Check sheet for the modelled part. Datum: model origin and axes. Units: mm. A direction names the side the tool comes from. Give positions to 0.01 mm unless a question says otherwise; leave off trailing zeros. Loops run counter-clockwise (first coordinate to the right, second up) from the corner with the lowest first, then second, coordinate; pieces in that order, holes last. Notation, with made-up numbers: M 80.5,7 L 119.5,7 A7 ccw 119.5,13 Z; hole C -15.5,76.25 d4. An arc over 180 degrees is marked long. Write each question's results on one line, items separated by ' | '. Start each with the question number.
1. Draft check along Y on faces 4 (the flat face through (59, 0, -65)), 5 (the cylindrical face through (149.01, 18.7, -107.05)), 6 (the flat face through (0, 12, -17)). Enter one of: pulls with the +Y half, pulls with the -Y half, needs draft (parallel to the pull), parting line crosses it, or undercut.
2. Sectioned sample at D-D on z = -110. Record the cut outline in (x, y).
3. Tool access check on faces 1 (the flat face through (148, 20, -90)), 2 (the flat face through (-2, 17, -10)), 3 (the flat face through (75, 1, -60)). Record the directions out of +Z, -Z, +X, -X, +Y, -Y that give a thin tool (end or side, any length) a straight path to the whole face; none if there is none.
4. Go/stop test with flat-tipped pins: pin 1 (2 mm diameter, centred on y = 16, z = -93, fed in from -X); pin 2 (2 mm diameter, centred on x = 28.5, y = 1, fed in from -Z); pin 3 (2 mm diameter, centred on y = 5.5, z = -97, fed in from -X); pin 4 (0.6 mm diameter, centred on x = -1, y = 17, fed in from -Z). Record where each tip stops, or that it passes through.
5. Sectioned sample at B-B on y = 16. Record the cut outline in (x, z), and give its area (3 significant figures).
6. Sectioned sample at A-A on z = -77. Record the cut outline in (x, y).
7. Sectioned sample at C-C on y = 4. Record the cut outline in (x, z), and give its area (3 significant figures).
8. Material ranges on line 1 along Y through (x, z) = (149.15, -85); line 2 along Y through (x, z) = (148.8, -110); line 3 along Y through (x, z) = (149.6, -93), recorded low to high.
```python
from build123d import *

# Parameters (mm, degrees)
BOSS_EXTRUDE1_DEPTH = 2
SKETCH2_W           = 2
SKETCH2_H           = 20
SKETCH2_H_2         = 60
BOSS_EXTRUDE2_DEPTH = 30
CUT_EXTRUDE1_REACH  = 212.533
SKETCH3_R           = 5
SKETCH3_R_2         = 1.75
SKETCH3_R_3         = 4


with BuildPart() as part:
    # Sketch1 → Boss-Extrude1 (new body)
    with BuildSketch(Plane(origin=(0, 0, 0), x_dir=(1, 0, 0), z_dir=(0, 1, 0))):
        Polygon((150, 120), (150, 60), (0, 60), (0, 0), (-20, 0), (-20, 80), (130, 80), (130, 120), align=None)
    extrude(amount=BOSS_EXTRUDE1_DEPTH)

    # Sketch2 → Boss-Extrude2 (add)
    with BuildSketch(Plane(origin=(0, 2, 0), x_dir=(1, 0, 0), z_dir=(0, 1, 0))):
        with Locations((-19, 10)):
            Rectangle(SKETCH2_W, SKETCH2_H)
        with Locations((-1, 10)):
            Rectangle(SKETCH2_W, SKETCH2_H)
        with Locations((149, 90)):
            Rectangle(SKETCH2_W, SKETCH2_H_2)
    extrude(amount=BOSS_EXTRUDE2_DEPTH)

    # Sketch3 → Cut-Extrude1 (cut, up to next)
    with BuildSketch(Plane(origin=(150, 0, 0), x_dir=(0, 0, -1), z_dir=(1, 0, 0)), mode=Mode.PRIVATE) as cut_extrude1_sk1:
        with Locations((85, 16)):
            Circle(SKETCH3_R)
    cut_extrude1_tool1 = extrude(cut_extrude1_sk1.sketch, amount=-CUT_EXTRUDE1_REACH, mode=Mode.PRIVATE) & part.part
    # Sketch3 → Cut-Extrude1 (cut, up to next)
    with BuildSketch(Plane(origin=(150, 0, 0), x_dir=(0, 0, -1), z_dir=(1, 0, 0)), mode=Mode.PRIVATE) as cut_extrude1_sk2:
        with Locations((85, 24)):
            Circle(SKETCH3_R_2)
    cut_extrude1_tool2 = extrude(cut_extrude1_sk2.sketch, amount=-CUT_EXTRUDE1_REACH, mode=Mode.PRIVATE) & part.part
    # Sketch3 → Cut-Extrude1 (cut, up to next)
    with BuildSketch(Plane(origin=(150, 0, 0), x_dir=(0, 0, -1), z_dir=(1, 0, 0)), mode=Mode.PRIVATE) as cut_extrude1_sk3:
        with Locations((93, 16)):
            Circle(SKETCH3_R_2)
    cut_extrude1_tool3 = extrude(cut_extrude1_sk3.sketch, amount=-CUT_EXTRUDE1_REACH, mode=Mode.PRIVATE) & part.part
    # Sketch3 → Cut-Extrude1 (cut, up to next)
    with BuildSketch(Plane(origin=(150, 0, 0), x_dir=(0, 0, -1), z_dir=(1, 0, 0)), mode=Mode.PRIVATE) as cut_extrude1_sk4:
        with Locations((85, 8)):
            Circle(SKETCH3_R_2)
    cut_extrude1_tool4 = extrude(cut_extrude1_sk4.sketch, amount=-CUT_EXTRUDE1_REACH, mode=Mode.PRIVATE) & part.part
    # Sketch3 → Cut-Extrude1 (cut, up to next)
    with BuildSketch(Plane(origin=(150, 0, 0), x_dir=(0, 0, -1), z_dir=(1, 0, 0)), mode=Mode.PRIVATE) as cut_extrude1_sk5:
        with Locations((77, 16)):
            Circle(SKETCH3_R_2)
    cut_extrude1_tool5 = extrude(cut_extrude1_sk5.sketch, amount=-CUT_EXTRUDE1_REACH, mode=Mode.PRIVATE) & part.part
    # Sketch3 → Cut-Extrude1 (cut, up to next)
    with BuildSketch(Plane(origin=(150, 0, 0), x_dir=(0, 0, -1), z_dir=(1, 0, 0)), mode=Mode.PRIVATE) as cut_extrude1_sk6:
        with Locations((110, 16)):
            Circle(SKETCH3_R_3)
    cut_extrude1_tool6 = extrude(cut_extrude1_sk6.sketch, amount=-CUT_EXTRUDE1_REACH, mode=Mode.PRIVATE) & part.part
    add(cut_extrude1_tool1.solids().sort_by_distance((150, 16, -85))[0], mode=Mode.SUBTRACT)
    add(cut_extrude1_tool2.solids().sort_by_distance((150, 24, -85))[0], mode=Mode.SUBTRACT)
    add(cut_extrude1_tool3.solids().sort_by_distance((150, 16, -93))[0], mode=Mode.SUBTRACT)
    add(cut_extrude1_tool4.solids().sort_by_distance((150, 8, -85))[0], mode=Mode.SUBTRACT)
    add(cut_extrude1_tool5.solids().sort_by_distance((150, 16, -77))[0], mode=Mode.SUBTRACT)
    add(cut_extrude1_tool6.solids().sort_by_distance((150, 16, -110))[0], mode=Mode.SUBTRACT)


solid = part.part
```
Output values:
1) face 4: pulls with the -Y half | face 5: undercut | face 6: needs draft
2) outline: M 130,0 L 150,0 L 150,12 L 148,12 L 148,2 L 130,2 Z; M 148,20 L 150,20 L 150,32 L 148,32 Z
3) face 1: +Z, -Z, -X, +Y | face 2: +Z, -Z, +Y | face 3: +Z, +X, +Y, -Y
4) pin 1: through | pin 2: z = -80 | pin 3: x = 148 | pin 4: z = -20
5) outline: M -20,-20 L -18,-20 L -18,0 L -20,0 Z; M -2,-20 L 0,-20 L 0,0 L -2,0 Z; M 148,-120 L 150,-120 L 150,-114 L 148,-114 Z; M 148,-106 L 150,-106 L 150,-94.75 L 148,-94.75 Z; M 148,-91.25 L 150,-91.25 L 150,-90 L 148,-90 Z; M 148,-80 L 150,-80 L 150,-78.75 L 148,-78.75 Z; M 148,-75.25 L 150,-75.25 L 150,-60 L 148,-60 Z | area: 150 mm2
6) outline: M -20,0 L 150,0 L 150,14.25 L 148,14.25 L 148,2 L -20,2 Z; M 148,17.75 L 150,17.75 L 150,32 L 148,32 Z
7) outline: M -20,-20 L -18,-20 L -18,0 L -20,0 Z; M -2,-20 L 0,-20 L 0,0 L -2,0 Z; M 148,-120 L 150,-120 L 150,-60 L 148,-60 Z | area: 200 mm2
8) line 1: 0 to 6.25, 9.75 to 11, 21 to 22.25, 25.75 to 32 | line 2: 0 to 12, 20 to 32 | line 3: 0 to 14.25, 17.75 to 32
